For this review, use the dimensioned drawing (mm, ordinates from the lowest corner) and the shaded views. A direction names the side the tool comes from. Coordinates: 2 decimals unless noted, no trailing zeros. Loops run counter-clockwise (first coordinate to the right, second up) from the corner with the lowest first, then second, coordinate; pieces in that order, holes last. Notation, with made-up numbers: (80.5, 82) - (134.5, 82) arc R14 ccw to (134.5, 108) - close; hole circle Ø4 at (9, 42). An arc over 180 degrees is marked (long way). Answer in a Markdown table with one row per item. Add a question column.
(1) For the marked faces 1 and 2, list the 3-axis set-ups (+Z, -Z, +X, -X, +Y, -Y) from which the entire face can be reached by the end or side of a thin tool; tool diameter is ignored.
(2) We need section C-C, the plane x = 52. Write out the cut boundary in (y, z).
(3) To check wall thickness, follow L1, parallel to X at y = 10, z = 31; L2, parallel to X at y = 6.75, z = 79; L3, parallel to Z at x = 54.5, y = 16.5. State the ranges of each line that lie inside material, in increasing order. Write a range as [from, to].
(4) Clearance check with flat-ended pins moving along their axes: pin 1 (6 mm diameter, centred on x = 31.5, y = 8.5, fed in from -Z); pin 2 (6 mm diameter, centred on y = 15, z = 9, fed in from +X). State where each tip first meets the part, or that it passes through.
(5) We need section B-B, the plane z = 31. Write out the cut boundary in (x, y), plus the area to 3 significant figures.
(6) We need section D-D, the plane z = 79. Write out the cut boundary in (x, y).
(7) We need section A-A, the plane x = 4. Write out the cut boundary in (y, z).
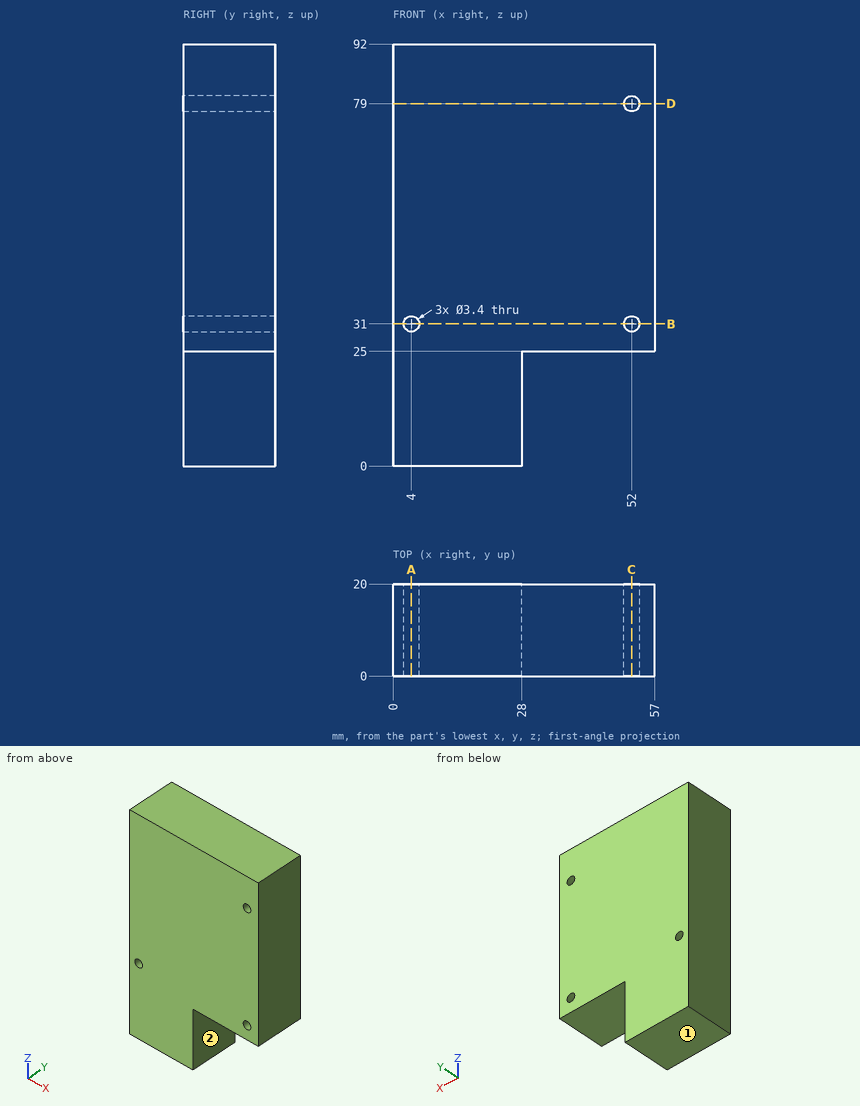
Responses:
| question | item | result |
|---|---|---|
| 1 | face 1 | -Z, +X, -X, +Y, -Y |
| 1 | face 2 | -Z, +X, +Y, -Y |
| 2 | outline | (0, 25) - (20, 25) - (20, 29.3) - (0, 29.3) - close; (0, 32.7) - (20, 32.7) - (20, 77.3) - (0, 77.3) - close; (0, 80.7) - (20, 80.7) - (20, 92) - (0, 92) - close |
| 3 | L1 | x = [0, 2.3], [5.7, 50.3], [53.7, 57] |
| 3 | L2 | x = [0, 50.3], [53.7, 57] |
| 3 | L3 | z = [25, 92] |
| 4 | pin 1 | stops at z = 25 |
| 4 | pin 2 | stops at x = 28 |
| 5 | outline | (0, 0) - (2.3, 0) - (2.3, 20) - (0, 20) - close; (5.7, 0) - (50.3, 0) - (50.3, 20) - (5.7, 20) - close; (53.7, 0) - (57, 0) - (57, 20) - (53.7, 20) - close |
| 5 | area | 1,000 mm2 |
| 6 | outline | (0, 0) - (50.3, 0) - (50.3, 20) - (0, 20) - close; (53.7, 0) - (57, 0) - (57, 20) - (53.7, 20) - close |
| 7 | outline | (0, 0) - (20, 0) - (20, 29.3) - (0, 29.3) - close; (0, 32.7) - (20, 32.7) - (20, 92) - (0, 92) - close |
